```python
from build123d import *

# Parameters (mm, degrees)
F0_W            = 40
F0_H            = 15
F1_DEPTH        = 12
F3_DEPTH        = 8
F5_DEPTH        = 4
F6_W            = 1.5
F6_H            = 3.5
F7_DEPTH        = 15
F8_W            = 0.5
F8_H            = 3.5
F8_W_2          = 29.5
F9_DEPTH        = 15
F11_D           = 3.4
F11_CBORE_D     = 6.5
F11_CBORE_DEPTH = 3


# Not quite as in the source:
# - a pattern or mirror of a feature is missing from the dataset's text; its kind, count and spacing are read off the source's solid


with BuildPart() as f1:
    # F0 (on Top) → F1 (new body)
    with BuildSketch(Plane.XY):
        with Locations((0, -7.5)):
            Rectangle(F0_W, F0_H)
    extrude(amount=F1_DEPTH)

    # F2 (on face) → F3 (cut)
    with BuildSketch(Plane.XY.offset(12)):
        with BuildLine():
            Line((-14.5, -15), (14.5, -15))
            ThreePointArc((14.5, -15), (0, -0.5), (-14.5, -15))
        make_face()
    extrude(amount=-F3_DEPTH, mode=Mode.SUBTRACT)

    # F4 (on face) → F5 (cut, through all)
    with BuildSketch(Plane.XY.offset(4)):
        with BuildLine():
            Line((-12, -15), (12, -15))
            ThreePointArc((12, -15), (0, -3), (-12, -15))
        make_face()
    extrude(amount=-F5_DEPTH, mode=Mode.SUBTRACT)

    # F6 (on face) → F7 (cut, through all)
    with BuildSketch(Plane.XZ.offset(15)):
        with Locations((-19.25, 10.25)):
            Rectangle(F6_W, F6_H)
    f7 = extrude(amount=-F7_DEPTH, mode=Mode.SUBTRACT)

    # F7_copies: F7 across plane
    add(f7.mirror(Plane(origin=(0, 0, 0), x_dir=(0, 0, 1), z_dir=(1, 0, 0))), mode=Mode.SUBTRACT)

    # F8 (on face) → F9 (cut, through all)
    with BuildSketch(Plane.XZ.offset(15)):
        with Locations((-14.75, 10.25)):
            Rectangle(F8_W, F8_H)
        with Locations((0.25, 10.25)):
            Rectangle(F8_W_2, F8_H)
    extrude(amount=-F9_DEPTH, mode=Mode.SUBTRACT)

    # F11 (through all)
    with Locations(Plane(origin=(0, 0, 0), x_dir=(-1, 0, 0), z_dir=(0, 1, 0))):
        with Locations((-16.5, 3.5)):
            f11 = CounterBoreHole(F11_D / 2, F11_CBORE_D / 2, F11_CBORE_DEPTH)

    # F11_copies: F11 across plane
    add(f11.mirror(Plane(origin=(0, 0, 0), x_dir=(0, 0, -1), z_dir=(-1, 0, 0))), mode=Mode.SUBTRACT)


solid = f1.part
```
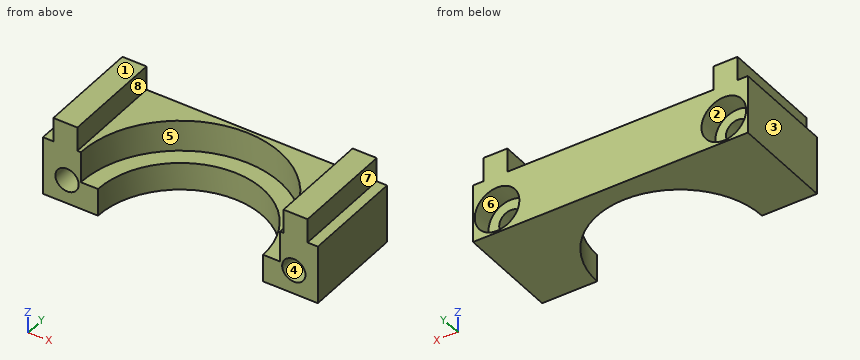
Source: CAD feature listing. Evaluate the final solid. Frame: model axes, mm. Face numbers are marked on the shaded views. A direction names the side the tool comes from. Give positions to 0.01 mm unless a question says otherwise; leave off trailing zeros. Loops run counter-clockwise (first coordinate to the right, second up) from the corner with the lowest first, then second, coordinate; pieces in that order, holes last. Notation, with made-up numbers: M -16.5,22.5 L 14.5,22.5 A17 ccw 14.5,26.5 Z; hole C -17,69 d1. An arc over 180 degrees is marked long. Put each result on its own line as item: value.
Q1. Section B-B (y = -12). Return the cut outline in (x, z), and give its area (3 significant figures).
Response values:
outline: M -20,0 L -11.62,0 L -11.62,4 L -14.19,4 L -14.19,8.5 L -15,8.5 L -15,12 L -18.5,12 L -18.5,8.5 L -20,8.5 Z; M 11.62,0 L 20,0 L 20,8.5 L 18.5,8.5 L 18.5,12 L 15,12 L 15,8.5 L 14.19,8.5 L 14.19,4 L 11.62,4 Z; hole C -16.5,3.5 d3.4; hole C 16.5,3.5 d3.4
area: 126 mm²
Q2. Mould query, pull axis Z, two halves, no side actions, for the marked faces 1, 2, 3 and 4. Classes: released by +Z, released by -Z, zero draft, split by the parting line, or undercut.
Response values:
face 1: released by +Z
face 2: undercut
face 3: zero draft
face 4: undercut
Q3. Section D-D (z = 3.5). Return the cut outline in (x, y), and give its area (3 significant figures).
Response values:
outline: M -20,-15 L -18.2,-15 L -18.2,-3 L -19.75,-3 L -19.75,0 L -20,0 Z; M -14.8,-15 L -12,-15 A12 cw 12,-15 L 14.8,-15 L 14.8,-3 L 13.25,-3 L 13.25,0 L -13.25,0 L -13.25,-3 L -14.8,-3 Z; M 18.2,-15 L 20,-15 L 20,0 L 19.75,0 L 19.75,-3 L 18.2,-3 Z
area: 253 mm²
Q4. Reachability of the marked faces 5, 6, 7 and 8 from +Z, -Z, +X, -X, +Y, -Y: full face, straight path, thin tool, end or side. Return the list, or none.
Response values:
face 5: +Z, -Y
face 6: +Y
face 7: +Z, +X, +Y, -Y
face 8: +Z, +Y, -Y
Q5. Pin query (flat end, axial travel): P1, Ø6, axis at x = -15, z = 2, coming from the +Y side; P2, Ø6, axis at x = -16.5, z = 3.5, coming from the +Y side; P3, Ø4, axis at y = -9, z = 11, coming from the -X side; P4, Ø2, axis at x = -4, z = 9, coming from the -Y side. Return the tip coordinate at first contact, or that it passes through.
Response values:
P1: stops at y = 0
P2: stops at y = -3
P3: stops at x = -18.5
P4: stops at y = -1.34
Q6. Line query: probe 1 along Z at (x, y) = (-16.5, -6.75); probe 2 along X at (y, z) = (-4.75, 9.25); probe 3 along X at (y, z) = (-13.5, 4.75). Output: solid intervals per line, ascending. Write a range as [from, to].
Response values:
probe 1: z = [0, 1.8], [5.2, 12]
probe 2: x = [-18.5, -15], [15, 18.5]
probe 3: x = [-20, -17.65], [-15.35, -14.42], [14.42, 15.35], [17.65, 20]
Q7. Section C-C (z = 10.5). Return the cut outline in (x, y), and give its area (3 significant figures).
Response values:
outline: M -18.5,-15 L -15,-15 L -15,0 L -18.5,0 Z; M 15,-15 L 18.5,-15 L 18.5,0 L 15,0 Z
area: 105 mm²
Q8. Section A-A (x = 16.5). Return the cut outline in (y, z), and give its area (3 significant figures).
Response values:
outline: M -15,0 L 0,0 L 0,0.25 L -3,0.25 L -3,1.8 L -15,1.8 Z; M -15,5.2 L -3,5.2 L -3,6.75 L 0,6.75 L 0,12 L -15,12 Z
area: 120 mm²
